Geometry check sheet. Reference: the model listing, model coordinates, mm. A direction names the side the tool comes from. Coordinates: 2 decimals unless noted, no trailing zeros. Write each loop counter-clockwise with the first axis right and the second up, starting at its lowest first coordinate (ties: lowest second). Pieces come first, ordered by that corner, then holes. Notation, with made-up numbers: M 4,-7.5 L 60,-7.5 A14 cw 60,13.5 Z; hole C -15.5,24 d5. An arc over 180 degrees is marked long. Answer as a JSON object with one key per item and string values. Group by question number.
```python
from build123d import *

# Parameters (mm, degrees)
BOSS_EXTRU_1_DEPTH      = 5
ESQUISSE2_W             = 11.095305832
ESQUISSE2_H             = 52.844950213
ESQUISSE2_W_2           = 7.610241821
ESQUISSE2_H_2           = 54.125177809
ENL_V_MAT_EXTRU_1_DEPTH = 10
ENL_V_MAT_EXTRU_2_DEPTH = 10


with BuildPart() as part:
    # Esquisse1 → Boss.-Extru.1 (new body)
    with BuildSketch(Plane.XY):
        Polygon((-12.911051911, 41.325067336), (-12.911051911, -8.174932664), (-6.211051911, -8.174932664), (-6.211051911, -3.174932664), (-4.511051911, -3.174932664), (-4.511051911, -1.178236629), (-5.761051911, -1.178236629), (-5.761051911, 1.821763371), (-4.511051911, 1.821763371), (-4.511051911, 9.575067336), (-1.311051911, 9.575067336), (-1.311051911, 1.821763371), (-0.061051911, 1.821763371), (-0.061051911, -1.178236629), (-1.311051911, -1.178236629), (-1.311051911, -3.174932664), (0.388948089, -3.174932664), (0.388948089, -8.174932664), (7.088948089, -8.174932664), (7.088948089, 41.325067336), (0.388948089, 41.325067336), (0.388948089, 36.325067336), (-1.311051911, 36.325067336), (-1.311051911, 34.328371301), (-0.061051911, 34.328371301), (-0.061051911, 31.328371301), (-1.311051911, 31.328371301), (-1.311051911, 23.575067336), (-4.511051911, 23.575067336), (-4.511051911, 31.328371301), (-5.761051911, 31.328371301), (-5.761051911, 34.328371301), (-4.511051911, 34.328371301), (-4.511051911, 36.325067336), (-6.211051911, 36.325067336), (-6.211051911, 41.325067336), align=None)
    extrude(amount=BOSS_EXTRU_1_DEPTH)

    # Esquisse2 → Enlèv. mat.-Extru.1 (cut)
    with BuildSketch(Plane(origin=(0, 0, 0), x_dir=(-1, 0, 0), z_dir=(0, 0, -1))):
        with Locations((-10.136601005, 16.610629213)):
            Rectangle(ESQUISSE2_W, ESQUISSE2_H)
        with Locations((14.216172822, 16.610629214)):
            Rectangle(ESQUISSE2_W_2, ESQUISSE2_H_2)
    extrude(amount=-ENL_V_MAT_EXTRU_1_DEPTH, mode=Mode.SUBTRACT)

    # Esquisse3 → Enlèv. mat.-Extru.2 (cut)
    with BuildSketch(Plane(origin=(0, 0, 0), x_dir=(-1, 0, 0), z_dir=(0, 0, -1))):
        Polygon((5.220452988, 12.575067336), (7.529854064, 16.575067336), (5.220452988, 20.575067336), (0.601650834, 20.575067336), (-1.707750243, 16.575067336), (0.601650834, 12.575067336), align=None)
    extrude(amount=-ENL_V_MAT_EXTRU_2_DEPTH, mode=Mode.SUBTRACT)


solid = part.part
```
1) Section check B-B (x = -2). Record the cut outline in (y, z).
2) Section check A-A (y = -4). Record the cut outline in (x, z).
3) Set-up check for faces 4 (the flat face through (-3, 9.575, 2)), 5 (the flat face through (-8, 17, 0)), 6 (the flat face through (-5, 1.822, 2)), 7 (the flat face through (0.389, 39, 2)): record each of +Z, -Z, +X, -X, +Y, -Y from which the full face is reachable in a straight line by a thin tool's end or side.
4) Material ranges on probe 1 along X at (y, z) = (33, 2.35); probe 2 along X at (y, z) = (38, 3.5); probe 3 along Y at (x, z) = (-0.25, 1.7), recorded low to high. Write a range as [from, to].
5) Go/stop test with flat-tipped pins: pin 1 Ø1.4 at (x, z) = (-5, 2.5) entering from -Y; pin 2 Ø0.5 at (x, z) = (0, 3.5) entering from +Y. Record where each tip stops, or that it passes through.
6) Draft check along X on faces 1 (the flat face through (4.589, 16, 2)), 2 (the flat face through (2, -8.175, 2)), 3 (the flat face through (-6.211, 39, 2)). Enter one of: +X half, -X half, draft (parallel to the pull), parting line (faces both ways), or undercut.
Entries:
{
 "1": {"outline": "M 9.58,0 L 12.58,0 L 12.58,5 L 9.58,5 Z; M 20.58,0 L 23.58,0 L 23.58,5 L 20.58,5 Z"},
 "2": {"outline": "M -10.41,0 L -6.21,0 L -6.21,5 L -10.41,5 Z; M 0.39,0 L 4.59,0 L 4.59,5 L 0.39,5 Z"},
 "3": {"face 4": "+Z, -Z, -Y", "face 5": "-Z, +X, -X, +Y, -Y", "face 6": "+Z, -Z", "face 7": "+Z, -Z, +Y"},
 "4": {"probe 1": "[-10.41, -5.76], [-0.06, 4.59]", "probe 2": "[-10.41, -6.21], [0.39, 4.59]", "probe 3": "[-3.17, -1.18], [1.82, 13.18], [19.97, 31.33], [34.33, 36.33]"},
 "5": {"pin 1": "y = -3.17", "pin 2": "y = 36.33"},
 "6": {"face 1": "+X half", "face 2": "draft", "face 3": "undercut"}
}
